from build123d import *

# Parameters (mm, degrees)
SKETCH_1_R               = 44.95
SKETCH_1_R_2             = 2.1
SKETCH_1_R_3             = 18.4
EXTRUDE_1_DEPTH          = 16
SKETCH_2_R               = 4
CUT_EXTRUDE_1_DEPTH      = 3
SKETCH_4_R               = 4.5
CUT_EXTRUDE_2_DEPTH      = 5.1
SKETCH_5_R               = 1.25
CUT_EXTRUDE_3_DEPTH      = 10
PATTERN_CIRCULAR_1_COUNT = 12
FILLET_1_R               = 0.5


with BuildPart() as part:
    # 草图1 → 凸台-拉伸1 (new body)
    with BuildSketch(Plane(origin=(0, 0, 0), x_dir=(1, 0, 0), z_dir=(0, 1, 0))):
        Circle(SKETCH_1_R)
        with Locations((-24.6, 0)):
            Circle(SKETCH_1_R_2, mode=Mode.SUBTRACT)
        with Locations((-12.3, 21.304224933)):
            Circle(SKETCH_1_R_2, mode=Mode.SUBTRACT)
        with Locations((12.3, 21.304224933)):
            Circle(SKETCH_1_R_2, mode=Mode.SUBTRACT)
        with Locations((24.6, 0)):
            Circle(SKETCH_1_R_2, mode=Mode.SUBTRACT)
        with Locations((12.3, -21.304224933)):
            Circle(SKETCH_1_R_2, mode=Mode.SUBTRACT)
        with Locations((-12.3, -21.304224933)):
            Circle(SKETCH_1_R_2, mode=Mode.SUBTRACT)
        Circle(SKETCH_1_R_3, mode=Mode.SUBTRACT)
    extrude(amount=EXTRUDE_1_DEPTH)

    # 草图2 → 切除-拉伸1 (cut)
    with BuildSketch(Plane.XZ):
        with Locations((-21.304224933, -12.3)):
            Circle(SKETCH_2_R)
        with Locations((0, 24.6)):
            Circle(SKETCH_2_R)
        with Locations((21.304224933, -12.3)):
            Circle(SKETCH_2_R)
    extrude(amount=-CUT_EXTRUDE_1_DEPTH, mode=Mode.SUBTRACT)

    # 草图4 → 切除-拉伸2 (cut)
    with BuildSketch(Plane(origin=(0, 16, 0), x_dir=(1, 0, 0), z_dir=(0, 1, 0))):
        with Locations((-24.6, 0)):
            Circle(SKETCH_4_R)
        with Locations((-12.3, 21.304224933)):
            Circle(SKETCH_4_R)
        with Locations((12.3, 21.304224933)):
            Circle(SKETCH_4_R)
        with Locations((24.6, 0)):
            Circle(SKETCH_4_R)
        with Locations((12.3, -21.304224933)):
            Circle(SKETCH_4_R)
        with Locations((-12.3, -21.304224933)):
            Circle(SKETCH_4_R)
    extrude(amount=-CUT_EXTRUDE_2_DEPTH, mode=Mode.SUBTRACT)

    # 草图5 → 切除-拉伸3 (cut)
    with BuildSketch(Plane(origin=(45, 0, 0), x_dir=(0, 0, -1), z_dir=(1, 0, 0))):
        with Locations((0, 12)):
            Circle(SKETCH_5_R)
    cut_extrude_3 = extrude(amount=-CUT_EXTRUDE_3_DEPTH, mode=Mode.SUBTRACT)

    # 阵列(圆周)1: 切除-拉伸3 ×12 about axis
    pattern_circular_1_axis = Axis((0, 0, 0), (0, 1, 0))
    for i in range(1, PATTERN_CIRCULAR_1_COUNT):
        add(cut_extrude_3.rotate(pattern_circular_1_axis, i * 360 / PATTERN_CIRCULAR_1_COUNT), mode=Mode.SUBTRACT)

    # 圆角1
    fillet_1_edges = [part.edges().sort_by_distance(p)[0] for p in [
        (-18.4, 16, 0),
    ]]
    fillet(fillet_1_edges, radius=FILLET_1_R)


solid = part.part
Design review of the part built by this model. Coordinates are the model's own, in mm. A direction names the side the tool comes from. Round coordinates to 2 decimals unless told otherwise and drop trailing zeros. Write each loop counter-clockwise with the first axis right and the second up, starting at its lowest first coordinate (ties: lowest second). Pieces come first, ordered by that corner, then holes. Notation, with made-up numbers: (54, 12) -> (66, 12) arc R19 ccw to (66, 42) -> close; hole circle Ø6 at (77.25, 68.5). An arc over 180 degrees is marked (long way). One line per question, with ' | ' between items.
(1) Take a section at B-B, the plane z = 0. State how many separate pieces and enclosed holes the cut face has, and give its area (3 significant figures).
Result sheet:
separate pieces: 4 | enclosed holes: 0 | area: 616 mm2
(2) Insertion check: P1, Ø7, axis at x = -12.3, z = -21.3, coming from the +Y side; P2, Ø8, axis at x = 25, y = 9.5, coming from the -Z side; P3, Ø5, axis at x = -14.5, y = 6.5, coming from the -Z side. Each pin has a flat end and moves straight along its axis. Give the tip position at first contact, or say it passes through.
Result sheet:
P1: y = 10.9 | P2: z = -39.74 | P3: z = -43.32
(3) Take a section at A-A, the plane x = 0. State the section outline as (y, z) points, and give its area (3 significant figures).
Result sheet:
outline: (0, -44.95) -> (10.75, -44.95) -> (10.75, -35) -> (13.25, -35) -> (13.25, -44.95) -> (16, -44.95) -> (16, -18.9) arc R0.5 ccw to (15.5, -18.4) -> (0, -18.4) -> close; (0, 18.4) -> (15.5, 18.4) arc R0.5 ccw to (16, 18.9) -> (16, 44.95) -> (13.25, 44.95) -> (13.25, 35) -> (10.75, 35) -> (10.75, 44.95) -> (0, 44.95) -> (0, 28.6) -> (3, 28.6) -> (3, 20.6) -> (0, 20.6) -> close | area: 776 mm2
(4) Take a section at C-C, the plane y = 7.75. State the section outline as (x, z) points, and give its area (3 significant figures).
Result sheet:
outline: circle Ø89.9 at (0, 0); hole circle Ø4.2 at (-24.6, 0); hole circle Ø36.8 at (0, 0); hole circle Ø4.2 at (-12.3, -21.3); hole circle Ø4.2 at (-12.3, 21.3); hole circle Ø4.2 at (12.3, -21.3); hole circle Ø4.2 at (12.3, 21.3); hole circle Ø4.2 at (24.6, 0) | area: 5,200 mm2
(5) Draft analysis for pull direction X (two halves, no side actions). For faces 6 (the flat face through (-35, 12, 0)), 7 (the flat face through (35, 12, 0)), 8 (the cylindrical face through (-25.19, 13.49, -4.46)), state which applies: released by +X, released by -X, zero draft, split by the parting line, or undercut.
Result sheet:
face 6: released by -X | face 7: released by +X | face 8: undercut
(6) Machinability: for faces 1 (the flat face through (30.32, 12.018, -17.485)), 2 (the cylindrical face through (40.04, 13.24, 0.16)), 3 (the cylindrical face through (0.16, 13.24, -40.04)), 4 (the flat face through (0, 3, 25)), 5 (the flat face through (10, 10.9, 22)), which of the approach directions +Z, -Z, +X, -X, +Y, -Y give a long, thin tool a straight path to every point of the face, cutting with its end or side? Answer none if there is none.
Result sheet:
face 1: none | face 2: +X | face 3: -Z | face 4: -Y | face 5: +Y
(7) Wall thickness on line 1 (X direction, y = 7, z = 0); line 2 (X direction, y = 14.45, z = 0); line 3 (Y direction, x = 41, z = 0): over which ranges is each line inside the solid? List them lowest first. Write a range as [from, to].
Result sheet:
line 1: [-44.95, -26.7], [-22.5, -18.4], [18.4, 22.5], [26.7, 44.95] | line 2: [-44.95, -29.1], [-20.1, -18.4], [18.4, 20.1], [29.1, 44.95] | line 3: [0, 10.75], [13.25, 16]
